from build123d import *

# Parameters (mm, degrees)
F0_R     = 3
F1_DEPTH = 4
F3_DEPTH = 2
F4_R     = 2.5
F5_DEPTH = 42
F6_SIZE  = 0.5
F7_SIZE  = 0.2


with BuildPart() as f1:
    # F0 (on Top) → F1 (new body)
    with BuildSketch(Plane.XY):
        Circle(F0_R)
    extrude(amount=F1_DEPTH)

    # F2 (on face) → F3 (cut)
    with BuildSketch(Plane.XY.offset(4)):
        Polygon((2.5, -1.443376), (2.5, 1.443376), (0, 2.886751), (-2.5, 1.443376), (-2.5, -1.443376), (0, -2.886751), align=None)
    extrude(amount=-F3_DEPTH, mode=Mode.SUBTRACT)

    # F4 (on face) → F5 (join)
    with BuildSketch(Plane(origin=(0, 0, 0), x_dir=(1, 0, 0), z_dir=(0, 0, -1))):
        Circle(F4_R)
    extrude(amount=F5_DEPTH)

    # F6
    f6_edges = [f1.edges().sort_by_distance(p)[0] for p in [
        (-2.5, 0, -42),
    ]]
    chamfer(f6_edges, length=F6_SIZE)

    # F7
    f7_edges = [f1.edges().sort_by_distance(p)[0] for p in [
        (-3, 0, 0),
    ]]
    chamfer(f7_edges, length=F7_SIZE)


solid = f1.part
Here's how the part is built. I have some questions about the finished solid (model axes, mm). A direction names the side the tool comes from. Coordinates: 2 decimals unless noted, no trailing zeros. Order: outer loops, then holes, each group sorted by start corner. A loop starts at its lowest first (then second) coordinate and runs counter-clockwise, first axis right, second up.
Item 1: For faces 1 (the face through (-3, 0, 2)), 2 (the face through (1.233, -2.175, 3.014)), which set-ups out of +Z, -Z, +X, -X, +Y, -Y let a thin tool reach every point of the face, with its end or its side?
Result sheet:
face 1: +Z, -Z
face 2: +Z
Item 2: I need wall thicknesses on line 1 (Y direction, x = 0.1, z = -4); line 2 (Z direction, x = 0.3, y = -1.65); line 3 (X direction, y = -2.1, z = -6.5). Which ranges of each line are inside material? Lowest first, please.
Result sheet:
line 1: y = -2.5 to 2.5
line 2: z = -42 to 2
line 3: x = -1.36 to 1.36
Item 3: If we section it at A-A on y = 0: List the corners of the cut face in (x, z) for me.
Result sheet:
outline: (-3, 0.2) - (-2.8, 0) - (-2.5, 0) - (-2.5, -41.5) - (-2, -42) - (2, -42) - (2.5, -41.5) - (2.5, 0) - (2.8, 0) - (3, 0.2) - (3, 4) - (2.5, 4) - (2.5, 2) - (-2.5, 2) - (-2.5, 4) - (-3, 4) - close
Item 4: If we section it at B-B on z = -21: List the corners of the cut face in (x, y) for me.
Result sheet:
outline: circle Ø5 at (0, 0)
Item 5: If we mould it in two halves opening along X, with no side actions, what happens to faces 3 (the face through (2, 2, 4)), 4 (the face through (1.267, 2.155, 3.014)), 5 (the face through (-0.54, 2.44, -20.46))? For each: +X half, -X half, draft (parallel to the pull), parting line (faces both ways), or undercut.
Result sheet:
face 3: draft
face 4: undercut
face 5: parting line
Item 6: For P1, Ø2, axis at y = -0.5, z = 3, coming from the +X side; P2, Ø1, axis at x = 0.5, z = -17, coming from the +Y side; P3, Ø1, axis at y = -0.5, z = -15, coming from the +X side, each with a flat end and sliding along its axis, tell me the tip position at first contact or that it passes through.
Result sheet:
P1: stops at x = 3
P2: stops at y = 2.5
P3: stops at x = 2.5
